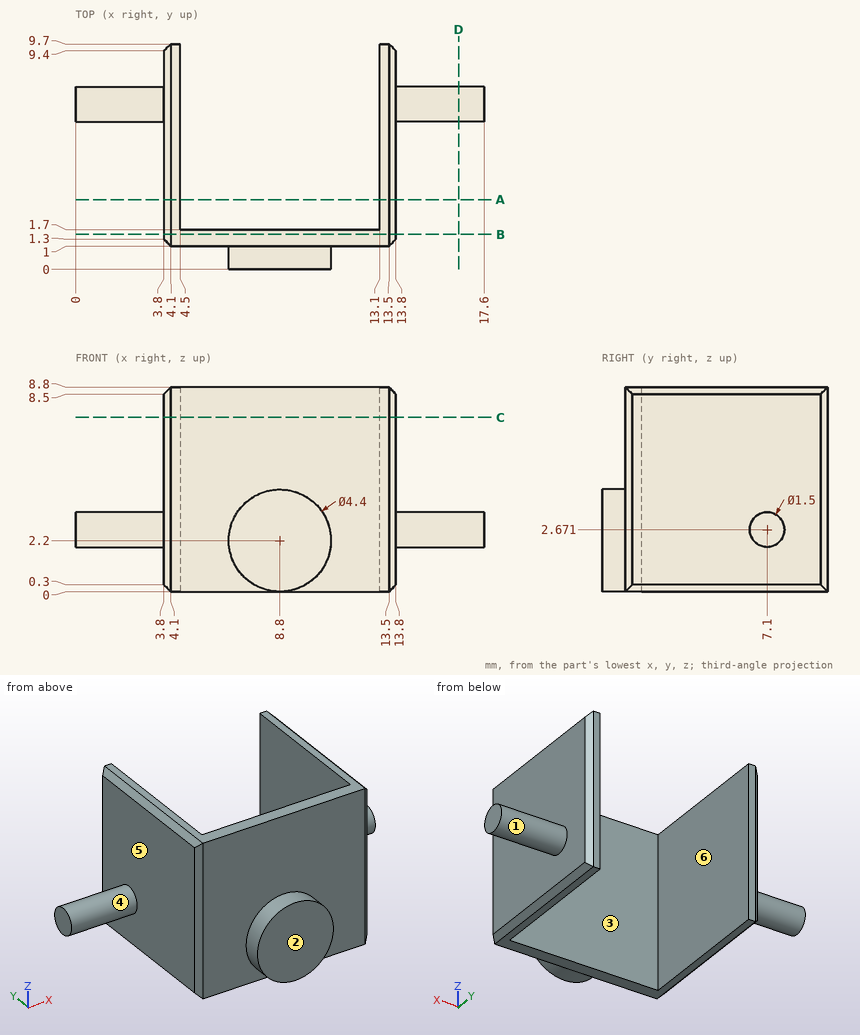
Verification items for this drawing (mm, ordinates from the low corner). A direction names the side the tool comes from. Give positions to 0.01 mm unless a question says otherwise; leave off trailing zeros. Write each loop counter-clockwise with the first axis right and the second up, starting at its lowest first coordinate (ties: lowest second). Pieces come first, ordered by that corner, then holes.
1) Gauge pin test, flat ends, axial feed: pin 1 (4 mm diameter, centred on y = 6, z = 6.5, fed in from -X); pin 2 (1 mm diameter, centred on x = 10.5, z = 7, fed in from +Y); pin 3 (1 mm diameter, centred on y = 3.5, z = 3.5, fed in from +X). Record the tip position at first contact, or that the pin passes through.
2) Section check B-B, the plane y = 1.5. Record the boundary of the cut face in (x, z).
3) Section check C-C, the plane z = 7.5. Record the boundary of the cut face in (x, y).
4) Release check for a two-part mould opening along X. For the marked faces 4, 5 and 6 record: pulls with the +X half, pulls with the -X half, needs draft (parallel to the pull), parting line crosses it, or undercut.
5) Section check D-D, the plane x = 16.5. Record the boundary of the cut face in (y, z).
6) Material ranges on L1, parallel to X at y = 2, z = 4.5; L2, parallel to Y at x = 11.5, z = 5.5; L3, parallel to Y at x = 9, z = 2, recorded low to high.
7) Section check A-A, the plane y = 3. Record the boundary of the cut face in (x, z).
8) Access from +Z, -Z, +X, -X, +Y, -Y to the whole of each face (thin tool, end or side, straight path). Record for the marked faces 1, 2 and 3.
Computed:
1. pin 1: stops at x = 3.8
1. pin 2: stops at y = 1.7
1. pin 3: stops at x = 13.8
2. outline: (3.8, 0.3) - (4.1, 0) - (13.5, 0) - (13.8, 0.3) - (13.8, 8.5) - (13.5, 8.8) - (4.1, 8.8) - (3.8, 8.5) - close
3. outline: (3.8, 1.3) - (4.1, 1) - (13.5, 1) - (13.8, 1.3) - (13.8, 9.4) - (13.5, 9.7) - (13.1, 9.7) - (13.1, 1.7) - (4.5, 1.7) - (4.5, 9.7) - (4.1, 9.7) - (3.8, 9.4) - close
4. face 4: needs draft
4. face 5: pulls with the -X half
4. face 6: undercut
5. outline: circle Ø1.5 at (7.1, 2.67)
6. L1: x = 3.8 to 4.5, 13.1 to 13.8
6. L2: y = 1 to 1.7
6. L3: y = 0 to 1.7
7. outline: (3.8, 0.3) - (4.1, 0) - (4.5, 0) - (4.5, 8.8) - (4.1, 8.8) - (3.8, 8.5) - close; (13.1, 0) - (13.5, 0) - (13.8, 0.3) - (13.8, 8.5) - (13.5, 8.8) - (13.1, 8.8) - close
8. face 1: +X
8. face 2: +Z, -Z, +X, -X, -Y
8. face 3: +Z, -Z, +Y
